The listing builds one solid part. Answer for the finished solid, in the listing's coordinates (mm). Face numbers are marked on the shaded views. A direction names the side the tool comes from. Round coordinates to 2 decimals unless told otherwise and drop trailing zeros. Write each loop counter-clockwise with the first axis right and the second up, starting at its lowest first coordinate (ties: lowest second). Pieces come first, ordered by that corner, then holes.
(1) A cutting plane is placed at D-D, the plane y = 59.5. Give the vertices of the cut face in (x, z), and give its area (3 significant figures).
(2) A cutting plane is placed at A-A, the plane z = 1.85. Give the vertices of the cut face in (x, y).
(3) Find the intervals of material crossed by probe 1 along Z at (x, y) = (-47.5, 43); probe 2 along X at (y, z) = (43, 1.4); probe 3 along Y at (x, z) = (-34, 1.05), in increasing order.
(4) The mould has two halves that part along X. Classify the marked faces 1 and 2: +X half, -X half, draft (parallel to the pull), parting line (faces both ways), or undercut.
(5) A cutting plane is placed at B-B, the plane y = 44. Give the vertices of the cut face in (x, z).
(6) A cutting plane is placed at C-C, the plane x = -43.5. Give the vertices of the cut face in (y, z), and give its area (3 significant figures).
(7) For the marked faces 3 and 4, determine the directions among +Z, -Z, +X, -X, +Y, -Y from which every point of the face is accessible in a straight line to the end or side of a thin tool.
from build123d import *

# Parameters (mm, degrees)
BOSS_EXTRUDE2_DEPTH = 5
CUT_EXTRUDE1_START  = 5
SKETCH3_W           = 19.008841094
SKETCH3_H           = 2.1
SKETCH3_W_2         = 12
SKETCH3_W_3         = 1.535533906
SKETCH3_W_4         = 1.464466094
SKETCH3_W_5         = 17.544375
CUT_EXTRUDE1_DEPTH  = 16
CUT_EXTRUDE2_DEPTH  = 52
SKETCH5_W           = 1.05
SKETCH5_H           = 46.149322856
CUT_EXTRUDE3_DEPTH  = 10
CUT_EXTRUDE4_START  = -0.76
CUT_EXTRUDE4_DEPTH  = 0.76
SKETCH7_W           = 2.828427125
SKETCH7_H           = 2.828427125
CUT_EXTRUDE5_DEPTH  = 0.1


with BuildPart() as part:
    # Sketch1 → Boss-Extrude2 (new body)
    with BuildSketch(Plane.XY):
        Polygon((-39.238867065, 47.72414844), (-47.72414844, 39.238867065), (-34.69381669, 26.208535316), (-26.208535316, 34.69381669), align=None)
        with BuildLine():
            ThreePointArc((-49.845468783, 62.573390845), (-56.568542495, 56.568542495), (-62.573390845, 49.845468783))
            Line((-62.573390845, 49.845468783), (-49.845468783, 37.117546722))
            Line((-49.845468783, 37.117546722), (-47.72414844, 39.238867065))
            Line((-47.72414844, 39.238867065), (-39.238867065, 47.72414844))
            Line((-39.238867065, 47.72414844), (-37.117546722, 49.845468783))
            Line((-37.117546722, 49.845468783), (-49.845468783, 62.573390845))
        make_face()
        with BuildLine():
            ThreePointArc((-34.594119865, 72.133534994), (-42.489529555, 67.783772971), (-49.845468783, 62.573390845))
            Line((-49.845468783, 62.573390845), (-37.117546722, 49.845468783))
            ThreePointArc((-37.117546722, 49.845468783), (-31.959737739, 60.548390845), (-34.594119865, 72.133534994))
        make_face()
        with BuildLine():
            ThreePointArc((-62.573390845, 49.845468783), (-67.783772971, 42.489529555), (-72.133534994, 34.594119865))
            ThreePointArc((-72.133534994, 34.594119865), (-60.548390845, 31.959737739), (-49.845468783, 37.117546722))
            Line((-49.845468783, 37.117546722), (-62.573390845, 49.845468783))
        make_face()
        with BuildLine():
            Line((-34.69381669, 26.208535316), (-35.779603128, 25.122748879))
            ThreePointArc((-35.779603128, 25.122748879), (-33.866185966, 25.503351216), (-32.244069222, 26.587214973))
            Line((-32.244069222, 26.587214973), (-26.587214973, 32.244069222))
            ThreePointArc((-26.587214973, 32.244069222), (-25.503351216, 33.866185966), (-25.122748879, 35.779603128))
            Line((-25.122748879, 35.779603128), (-26.208535316, 34.69381669))
            Line((-26.208535316, 34.69381669), (-34.69381669, 26.208535316))
        make_face()
    extrude(amount=BOSS_EXTRUDE2_DEPTH)

    # Sketch3 → Cut-Extrude1 (cut)
    with BuildSketch(Plane(origin=(-57.699913345, 57.699913345, 0), x_dir=(-0.707106781186549, -0.7071067811865461, 0), z_dir=(0.7071067811865461, -0.707106781186549, 0)).offset(CUT_EXTRUDE1_START)):
        with Locations((-17.039954453, -2.5)):
            Rectangle(SKETCH3_W, SKETCH3_H)
        with Locations((0, -2.5)):
            Rectangle(SKETCH3_W_2, SKETCH3_H)
        with Locations((-6.767766953, -2.5)):
            Rectangle(SKETCH3_W_3, SKETCH3_H)
        with Locations((6.767766953, -2.5)):
            Rectangle(SKETCH3_W_3, SKETCH3_H)
        with Locations((8.267766953, -2.5)):
            Rectangle(SKETCH3_W_4, SKETCH3_H)
        with Locations((17.7721875, -2.5)):
            Rectangle(SKETCH3_W_5, SKETCH3_H)
    extrude(amount=CUT_EXTRUDE1_DEPTH, mode=Mode.SUBTRACT)

    # Sketch4 → Cut-Extrude2 (cut)
    with BuildSketch(Plane(origin=(-57.699913345, 57.699913345, 0), x_dir=(-0.707106781186549, -0.7071067811865461, 0), z_dir=(0.7071067811865461, -0.707106781186549, 0))):
        Polygon((-7.535533906, -2.5), (27.054152634, -2.5), (27.054152634, -6.972921607), (-28.074504585, -6.972921607), (-28.074504585, -2.5), align=None)
    extrude(amount=CUT_EXTRUDE2_DEPTH, mode=Mode.SUBTRACT)

    # Sketch5 → Cut-Extrude3 (cut)
    with BuildSketch(Plane(origin=(-54.164379439, 54.164379439, 0), x_dir=(0, 0, -1), z_dir=(0.7071067811865461, -0.7071067811865489, 0))):
        with Locations((-1.975, 0)):
            Rectangle(SKETCH5_W, SKETCH5_H)
    extrude(amount=-CUT_EXTRUDE3_DEPTH, mode=Mode.SUBTRACT)

    # Sketch6 → Cut-Extrude4 (cut)
    with BuildSketch(Plane.XY.offset(1.45).offset(CUT_EXTRUDE4_START)):
        with BuildLine():
            Line((-47.72414844, 39.238867065), (-49.845468783, 37.117546722))
            ThreePointArc((-49.845468783, 37.117546722), (-60.548390845, 31.959737739), (-72.133534994, 34.594119865))
            ThreePointArc((-72.133534994, 34.594119865), (-56.568542495, 56.568542495), (-34.594119865, 72.133534994))
            ThreePointArc((-34.594119865, 72.133534994), (-31.959737739, 60.548390845), (-37.117546722, 49.845468783))
            Line((-37.117546722, 49.845468783), (-39.238867065, 47.72414844))
            Line((-39.238867065, 47.72414844), (-38.608030253, 47.093311627))
            Line((-38.608030253, 47.093311627), (-47.093311627, 38.608030253))
            Line((-47.093311627, 38.608030253), (-47.72414844, 39.238867065))
        make_face()
    extrude(amount=CUT_EXTRUDE4_DEPTH, mode=Mode.SUBTRACT)

    # Sketch7 → Cut-Extrude5 (cut)
    with BuildSketch(Plane.XY.offset(2.5)):
        with Locations((-35.355339059, 35.355339059)):
            Rectangle(SKETCH7_W, SKETCH7_H)
    extrude(amount=-CUT_EXTRUDE5_DEPTH, mode=Mode.SUBTRACT)


solid = part.part
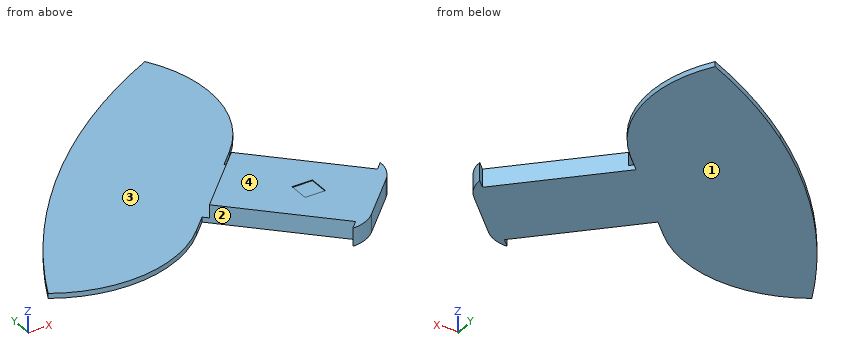
Solutions:
1. outline: (-53.48, 0) - (-32.11, 0) - (-32.11, 0.69) - (-53.48, 0.69) - close
1. area: 14.7 mm2
2. outline: (-47.09, 38.61) - (-34.69, 26.21) - (-35.78, 25.12) arc R5 ccw to (-32.24, 26.59) - (-26.59, 32.24) arc R5 ccw to (-25.12, 35.78) - (-26.21, 34.69) - (-38.61, 47.09) - close
3. probe 1: z = 0 to 0.69
3. probe 2: x = -42.7 to -34.51
3. probe 3: y = 25.45 to 42.49
4. face 1: draft
4. face 2: undercut
5. outline: (-66.81, 0) - (-35.51, 0) - (-35.51, 2.5) - (-41.7, 2.5) - (-41.7, 0.69) - (-66.81, 0.69) - close
6. outline: (35.01, 0) - (67.14, 0) - (67.14, 0.69) - (42.2, 0.69) - (42.2, 2.5) - (35.01, 2.5) - close
6. area: 35.2 mm2
7. face 3: +Z, -X, +Y
7. face 4: +Z, +X, -X, +Y, -Y
